Check sheet for the modelled part. Datum: model origin and axes. Units: mm. A direction names the side the tool comes from. Coordinates: 2 decimals unless noted, no trailing zeros. Loops run counter-clockwise (first coordinate to the right, second up) from the corner with the lowest first, then second, coordinate; pieces in that order, holes last. Notation, with made-up numbers: M 72.25,70.5 L 86.25,70.5 A18 ccw 86.25,103.5 Z; hole C 44,71 d6. An arc over 180 degrees is marked long. Answer in a Markdown table with one row per item. Add a question column.
```python
from build123d import *

# Parameters (mm, degrees)
CROQUIS2_W              = 131.1
CROQUIS2_H              = 54
SALIENTE_EXTRUIR2_DEPTH = 3
CROQUIS3_W              = 125.1
CROQUIS3_H              = 44
SALIENTE_EXTRUIR3_DEPTH = 34
CROQUIS4_W              = 131.1
CROQUIS4_H              = 37
SALIENTE_EXTRUIR4_DEPTH = 6.4
REDONDEO2_R             = 8.4


with BuildPart() as part:
    # Croquis2 → Saliente-Extruir2 (new body)
    with BuildSketch(Plane.XY):
        with Locations((65.55, -27)):
            Rectangle(CROQUIS2_W, CROQUIS2_H)
    extrude(amount=SALIENTE_EXTRUIR2_DEPTH)

    # Croquis3 → Saliente-Extruir3 (add)
    with BuildSketch(Plane.XY.offset(3)):
        Polygon((2, -6), (0, -6), (0, -54), (131.1, -54), (131.1, -6), (129.1, -6), (129.1, 0), (68.55, 0), (68.55, -6), (66.55, -6), (66.55, 0), (65.55, 0), (64.55, 0), (64.55, -6), (62.55, -6), (62.55, 0), (2, 0), align=None)
        with Locations((65.55, -29)):
            Rectangle(CROQUIS3_W, CROQUIS3_H, mode=Mode.SUBTRACT)
    extrude(amount=SALIENTE_EXTRUIR3_DEPTH)

    # Croquis4 → Saliente-Extruir4 (add)
    with BuildSketch(Plane.XZ.offset(54)):
        with Locations((65.55, 18.5)):
            Rectangle(CROQUIS4_W, CROQUIS4_H)
    extrude(amount=SALIENTE_EXTRUIR4_DEPTH)

    # Redondeo2
    redondeo2_edges = [part.edges().sort_by_distance(p)[0] for p in [
        (65.55, -60.4, 37),
    ]]
    fillet(redondeo2_edges, radius=REDONDEO2_R)


solid = part.part
```
Q1. Cross-section at D-D (z = 31.5). Record the cut outline in (x, y).
Q2. Thickness scan on L1, parallel to Y at x = 73.5, z = 19; L2, parallel to X at y = -20, z = 28; L3, parallel to Z at x = 41, y = -33. Record the ranges inside material, lowest first.
Q3. Cross-section at A-A (x = 123). Record the cut outline in (y, z).
Q4. Access from +Z, -Z, +X, -X, +Y, -Y to the whole of each face (thin tool, end or side, straight path). Record for faces 1 (the face through (65, -30, 0)), 2 (the face through (65, -60.4, 15)), 3 (the face through (2, -3, 20)), 4 (the face through (128.1, -29, 20)), 5 (the face through (66.55, -3, 20)).
Q5. Cross-section at C-C (z = 25). Record the cut outline in (x, y), plus the area to 3 significant figures.
Q6. Go/stop test with flat-tipped pins: pin 1 (1.6 mm diameter, centred on x = 130.5, z = 18, fed in from +Y); pin 2 (5 mm diameter, centred on y = -2, z = 21, fed in from -X); pin 3 (0.6 mm diameter, centred on x = 64, y = -2.5, fed in from +Z). Record where each tip stops, or that it passes through.
Q7. Mould release check, pull along Y, two halves, no side actions. Record for faces 6 (the face through (66.468, -57.874, 34.605)), 7 (the face through (3, -29, 20)), 8 (the face through (65, -29, 3)), 9 (the face through (129.1, -3, 20)): released by +Y, released by -Y, zero draft, split by the parting line, or undercut.
Q8. Cross-section at B-B (y = -8.5). Record the cut outline in (x, z).
Answer key:
| question | item | result |
|---|---|---|
| 1 | outline | M 0,-59.88 L 131.1,-59.88 L 131.1,-6 L 129.1,-6 L 129.1,0 L 68.55,0 L 68.55,-6 L 66.55,-6 L 66.55,0 L 64.55,0 L 64.55,-6 L 62.55,-6 L 62.55,0 L 2,0 L 2,-6 L 0,-6 Z; hole M 3,-51 L 128.1,-51 L 128.1,-7 L 3,-7 Z |
| 2 | L1 | -60.4 to -51, -7 to 0 |
| 2 | L2 | 0 to 3, 128.1 to 131.1 |
| 2 | L3 | 0 to 3 |
| 3 | outline | M -60.4,0 L 0,0 L 0,37 L -7,37 L -7,3 L -51,3 L -51,37 L -52,37 A8.4 ccw -60.4,28.6 Z |
| 4 | face 1 | -Z, +X, -X, +Y, -Y |
| 4 | face 2 | +Z, -Z, +X, -X, -Y |
| 4 | face 3 | +Z, -X, +Y |
| 4 | face 4 | +Z |
| 4 | face 5 | +Z, +Y |
| 5 | outline | M 0,-60.4 L 131.1,-60.4 L 131.1,-6 L 129.1,-6 L 129.1,0 L 68.55,0 L 68.55,-6 L 66.55,-6 L 66.55,0 L 64.55,0 L 64.55,-6 L 62.55,-6 L 62.55,0 L 2,0 L 2,-6 L 0,-6 Z; hole M 3,-51 L 128.1,-51 L 128.1,-7 L 3,-7 Z |
| 5 | area | 2,370 mm^2 |
| 6 | pin 1 | y = -6 |
| 6 | pin 2 | x = 2 |
| 6 | pin 3 | z = 3 |
| 7 | face 6 | released by -Y |
| 7 | face 7 | undercut |
| 7 | face 8 | undercut |
| 7 | face 9 | zero draft |
| 8 | outline | M 0,0 L 131.1,0 L 131.1,37 L 128.1,37 L 128.1,3 L 3,3 L 3,37 L 0,37 Z |
